Could you check a few things on this model? Use its own coordinates, in mm. Give positions to 0.01 mm unless a question says otherwise; leave off trailing zeros. Order: outer loops, then holes, each group sorted by start corner. A loop starts at its lowest first (then second) coordinate and runs counter-clockwise, first axis right, second up. Notation, with made-up numbers: (-36.75, 46) -> (-9.75, 46) arc R30 cw to (-9.75, 81) -> close; hole circle Ø10 at (39, 65.5). An arc over 180 degrees is marked (long way). Write each question's results on one line, items separated by ' | '.
```python
from build123d import *

# Parameters (mm, degrees)
SKETCH_R     = 25
SKETCH_R_2   = 21
SKETCH_R_3   = 19.584537
PAD_DEPTH    = 30
PAD001_DEPTH = 30


with BuildPart() as part:
    # Sketch → Pad (new body)
    with BuildSketch(Plane.XY):
        with BuildLine():
            Line((-35.584206, -63.111127), (44.415794, -63.111127))
            ThreePointArc((44.415794, -63.111127), (77.13309, -49.55918), (90.685038, -16.841884))
            Line((90.685038, -16.841884), (90.685038, 63.158116))
            ThreePointArc((90.685038, 63.158116), (77.13309, 95.875412), (44.415794, 109.427359))
            Line((44.415794, 109.427359), (-35.584206, 109.427359))
            ThreePointArc((-35.584206, 109.427359), (-68.301501, 95.875412), (-81.853449, 63.158116))
            Line((-81.853449, 63.158116), (-81.853449, -16.841884))
            ThreePointArc((-81.853449, -16.841884), (-68.301501, -49.55918), (-35.584206, -63.111127))
        make_face()
        with Locations((4.62833, 30.241158)):
            Circle(SKETCH_R, mode=Mode.SUBTRACT)
        with Locations((-50.106209, -31.898642)):
            Circle(SKETCH_R_2, mode=Mode.SUBTRACT)
        with Locations((59.362869, 78.858307)):
            Circle(SKETCH_R_3, mode=Mode.SUBTRACT)
    extrude(amount=PAD_DEPTH)

    # Sketch → Pad001 (join)
    with BuildSketch(Plane.XY):
        with BuildLine():
            Line((-35.584206, -63.111127), (44.415794, -63.111127))
            ThreePointArc((44.415794, -63.111127), (77.13309, -49.55918), (90.685038, -16.841884))
            Line((90.685038, -16.841884), (90.685038, 63.158116))
            ThreePointArc((90.685038, 63.158116), (77.13309, 95.875412), (44.415794, 109.427359))
            Line((44.415794, 109.427359), (-35.584206, 109.427359))
            ThreePointArc((-35.584206, 109.427359), (-68.301501, 95.875412), (-81.853449, 63.158116))
            Line((-81.853449, 63.158116), (-81.853449, -16.841884))
            ThreePointArc((-81.853449, -16.841884), (-68.301501, -49.55918), (-35.584206, -63.111127))
        make_face()
        with Locations((4.62833, 30.241158)):
            Circle(SKETCH_R, mode=Mode.SUBTRACT)
        with Locations((-50.106209, -31.898642)):
            Circle(SKETCH_R_2, mode=Mode.SUBTRACT)
        with Locations((59.362869, 78.858307)):
            Circle(SKETCH_R_3, mode=Mode.SUBTRACT)
    extrude(amount=PAD001_DEPTH)


solid = part.part
```
Q1. I need wall thicknesses on line 1 along X through (y, z) = (47, 26.5); line 2 along Y through (x, z) = (15, 22); line 3 along Y through (x, z) = (-47.5, 15.25). Which ranges of each line are inside material? Lowest first, please.
Here are the results:
line 1: x = -81.85 to -13.92, 23.18 to 90.69 | line 2: y = -63.11 to 7.49, 52.99 to 109.43 | line 3: y = -61.55 to -52.74, -11.06 to 107.87
Q2. Suppose I cut it at C-C on z = 17.25. Please give me the cut outline in (x, y), and give its area (3 significant figures).
Here are the results:
outline: (-81.85, -16.84) arc R46.27 ccw to (-35.58, -63.11) -> (44.42, -63.11) arc R46.27 ccw to (90.69, -16.84) -> (90.69, 63.16) arc R46.27 ccw to (44.42, 109.43) -> (-35.58, 109.43) arc R46.27 ccw to (-81.85, 63.16) -> close; hole circle Ø42 at (-50.11, -31.9); hole circle Ø50 at (4.63, 30.24); hole circle Ø39.17 at (59.36, 78.86) | area: 23,400 mm²
Q3. Thinking about a two-plate mould opening in X: for faces 1 (the flat face through (-81.853, 24, 15)), 2 (the flat face through (3, 5, 0)), 3 (the flat face through (90.685, 23, 15)), 4 (the cylindrical face through (18.1, 51.3, 14.8)), which applies, +X half, -X half, draft (parallel to the pull), parting line (faces both ways), or undercut?
Here are the results:
face 1: -X half | face 2: draft | face 3: +X half | face 4: undercut
Q4. Suppose I cut it at B-B on x = 1.5. Please give me the cut outline in (y, z), and give its area (3 significant figures).
Here are the results:
outline: (-63.11, 0) -> (5.44, 0) -> (5.44, 30) -> (-63.11, 30) -> close; (55.04, 0) -> (109.43, 0) -> (109.43, 30) -> (55.04, 30) -> close | area: 3,690 mm²
Q5. I'm going to push flat-ended pins straight in: pin 1 Ø8 at (x, y) = (-32.5, 12) entering from -Z; pin 2 Ø8 at (x, z) = (66.5, 10.5) entering from -Y; pin 3 Ø1 at (y, z) = (64, 22) entering from -X; pin 4 Ø1.5 at (x, z) = (73, 6) entering from +Y. Where does each tip first touch, or does it pass through?
Here are the results:
pin 1: stops at z = 0 | pin 2: stops at y = -59.43 | pin 3: stops at x = -81.85 | pin 4: stops at y = 100.12
Q6. Suppose I cut it at A-A on y = 68. Please give me the cut outline in (x, z), and give its area (3 significant figures).
Here are the results:
outline: (-81.6, 0) -> (43.06, 0) -> (43.06, 30) -> (-81.6, 30) -> close; (75.66, 0) -> (90.43, 0) -> (90.43, 30) -> (75.66, 30) -> close | area: 4,180 mm²
